from build123d import *

# Parameters (mm, degrees)
SKETCH1_R        = 16.8
BODY_DEPTH       = 11
BODYCHAMFER_SIZE = 0.5
BODYFLAT_START   = -6.35
BODYFLAT_DEPTH   = 6.35


with BuildPart() as part:
    # Sketch1 → Body (new body)
    with BuildSketch(Plane.XY):
        Circle(SKETCH1_R)
    extrude(amount=BODY_DEPTH)

    # BodyChamfer
    bodychamfer_edges = [part.edges().sort_by_distance(p)[0] for p in [
        (-16.8, 0, 11),
    ]]
    chamfer(bodychamfer_edges, length=BODYCHAMFER_SIZE)

    # Sketch2 → BodyFlat (cut)
    with BuildSketch(Plane.XY.offset(11).offset(BODYFLAT_START)):
        with BuildLine():
            Line((-13.462, -10.050599783), (-13.462, 10.050599783))
            ThreePointArc((-13.462, 10.050599783), (-16.8, 0), (-13.462, -10.050599783))
        make_face()
        with BuildLine():
            Line((13.462, -10.050599783), (13.462, 10.050599783))
            ThreePointArc((13.462, 10.050599783), (16.8, 0), (13.462, -10.050599783))
        make_face()
    extrude(amount=BODYFLAT_DEPTH, mode=Mode.SUBTRACT)

    # Sketch4 → 1/8 NPT Tapped Hole1 (revolve, cut)
    with BuildSketch(Plane(origin=(0, 0, 11), x_dir=(0, -1, 0), z_dir=(1, 0, 0))):
        Polygon((0, 0), (0, 14.533468714), (4.2164, 12), (4.2164, 7), (4.936183926, 7), (5.1457733, 0), align=None)
    revolve(axis=Axis((0, 0, 17.35), (0, 0, -1)), mode=Mode.SUBTRACT)


solid = part.part
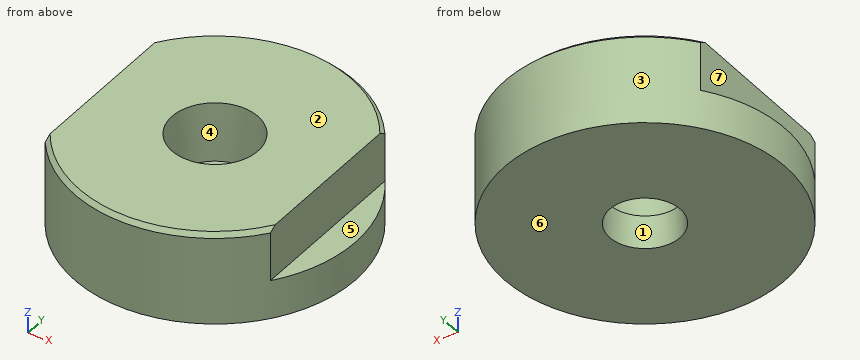
Here's how the part is built. I have some questions about the finished solid (model axes, mm). Face numbers are marked on the shaded views. A direction names the side the tool comes from. Give positions to 0.01 mm unless a question says otherwise; leave off trailing zeros. Loops run counter-clockwise (first coordinate to the right, second up) from the corner with the lowest first, then second, coordinate; pieces in that order, holes last. Notation, with made-up numbers: (51.5, 53.5) -> (93.5, 53.5) arc R13 cw to (93.5, 59.5) -> close; hole circle Ø10 at (4.25, 89.25). An arc over 180 degrees is marked (long way). One line per item, written item: value.
Q1. Suppose I cut it at D-D on z = 9.5. Please give me the cut outline in (x, y), then the cut area to 3 significant figures.
Answers follow:
outline: (-13.46, -10.05) arc R16.8 ccw to (13.46, -10.05) -> (13.46, 10.05) arc R16.8 ccw to (-13.46, 10.05) -> close; hole circle Ø10.2 at (0, 0)
area: 714 mm^2
Q2. Suppose I cut it at B-B on y = 0. Please give me the cut outline in (x, z).
Answers follow:
outline: (-16.8, 0) -> (-4.22, 0) -> (-4.22, 4) -> (-4.94, 4) -> (-5.15, 11) -> (-13.46, 11) -> (-13.46, 4.65) -> (-16.8, 4.65) -> close; (4.22, 0) -> (16.8, 0) -> (16.8, 4.65) -> (13.46, 4.65) -> (13.46, 11) -> (5.15, 11) -> (4.94, 4) -> (4.22, 4) -> close
Q3. I'm going to push flat-ended pins straight in: pin 1 Ø1 at (x, z) = (5.5, 8) entering from -Y; pin 2 Ø3 at (x, y) = (-1, 2) entering from +Z; pin 3 Ø1.9 at (y, z) = (0.5, 8.5) entering from -X; pin 4 Ø6 at (x, z) = (12, 2.5) entering from -Y. Where does each tip first touch, or does it pass through?
Answers follow:
pin 1: y = -16.04
pin 2: through
pin 3: x = -13.46
pin 4: y = -14.19
Q4. On a 3-axis mill with a long thin cutter (end or side, diameter ignored), from which of +Z, -Z, +X, -X, +Y, -Y can I reach the whole of each face in a straight line? I mean the marked faces 4, 5, 6 and 7. Say none if no direction works.
Answers follow:
face 4: +Z
face 5: +Z, +X, +Y, -Y
face 6: -Z, +X, -X, +Y, -Y
face 7: +Z, -X, +Y, -Y
Q5. We'd pull the mould along Y, two halves only. Please class the marked faces 1, 2 and 3: pulls with the +Y half, pulls with the -Y half, needs draft (parallel to the pull), parting line crosses it, or undercut.
Answers follow:
face 1: undercut
face 2: needs draft
face 3: parting line crosses it
Q6. If I drill on line 1 along Y through (x, z) = (0, 2.15); line 2 along X through (y, z) = (-8.5, 8), over which ranges is the centre line in solid material (lowest first)?
Answers follow:
line 1: -16.8 to -4.22, 4.22 to 16.8
line 2: -13.46 to 13.46
Q7. Suppose I cut it at C-C on z = 2.25. Please give me the cut outline in (x, y).
Answers follow:
outline: circle Ø33.6 at (0, 0); hole circle Ø8.43 at (0, 0)
Q8. Suppose I cut it at A-A on x = 0. Please give me the cut outline in (y, z), then the cut area to 3 significant figures.
Answers follow:
outline: (-16.8, 0) -> (-4.22, 0) -> (-4.22, 4) -> (-4.94, 4) -> (-5.15, 11) -> (-16.3, 11) -> (-16.8, 10.5) -> close; (4.22, 0) -> (16.8, 0) -> (16.8, 10.5) -> (16.3, 11) -> (5.15, 11) -> (4.94, 4) -> (4.22, 4) -> close
area: 265 mm^2
